Verification items for the finished model (mm, model axes). A direction names the side the tool comes from. Round coordinates to 2 decimals unless told otherwise and drop trailing zeros. Write each loop counter-clockwise with the first axis right and the second up, starting at its lowest first coordinate (ties: lowest second). Pieces come first, ordered by that corner, then holes. Notation, with made-up numbers: (89, 41.25) - (131, 41.25) arc R25 ccw to (131, 72.25) - close; hole circle Ø6 at (8.25, 53). An arc over 180 degrees is marked (long way). Write each question's results on one line, items separated by ' | '.
```python
from build123d import *

# Parameters (mm, degrees)
F0_R     = 5
F1_DEPTH = 78.5
F2_R     = 1.5
F3_DEPTH = 7


with BuildPart() as f1:
    # F0 (on Right) → F1 (new body)
    with BuildSketch(Plane.YZ):
        Circle(F0_R)
    extrude(amount=F1_DEPTH)

    # F2 (on face) → F3 (join)
    with BuildSketch(Plane.YZ.offset(78.5)):
        Circle(F2_R)
    extrude(amount=F3_DEPTH)

    # F4: F1 across plane


with BuildPart() as f1_1:
    add(f1.part)
    add(f1.part.mirror(Plane.YZ))


solid = f1_1.part
```
(1) Set-up check for faces 1 (the cylindrical face through (1.1, -1.08, -4.88)), 2 (the flat face through (78.5, -1.2, 1.2)), 3 (the cylindrical face through (-81.95, -1.5, 0.07)): record each of +Z, -Z, +X, -X, +Y, -Y from which the full face is reachable in a straight line by a thin tool's end or side.
Answer:
face 1: +X, -X | face 2: +X | face 3: -X
(2) Go/stop test with flat-tipped pins: pin 1 Ø2 at (x, z) = (19.5, 1.5) entering from -Y; pin 2 Ø1 at (x, y) = (-21, 3.5) entering from +Z; pin 3 Ø2 at (y, z) = (-0.5, 3.5) entering from +X. Record where each tip stops, or that it passes through.
Answer:
pin 1: y = -4.97 | pin 2: z = 4 | pin 3: x = 78.5
(3) Thickness scan on L1, parallel to Z at x = -5, y = 0.5; L2, parallel to X at y = -2, z = 1.5. Record the ranges inside material, lowest first.
Answer:
L1: -4.97 to 4.97 | L2: -78.5 to 78.5
(4) Section check A-A (z = 0). Record the cut outline in (x, y).
Answer:
outline: (-85.5, -1.5) - (-78.5, -1.5) - (-78.5, -5) - (78.5, -5) - (78.5, -1.5) - (85.5, -1.5) - (85.5, 1.5) - (78.5, 1.5) - (78.5, 5) - (-78.5, 5) - (-78.5, 1.5) - (-85.5, 1.5) - close
(5) Section check C-C (x = -3). Record the cut outline in (y, z), plus the area to 3 significant figures.
Answer:
outline: circle Ø10 at (0, 0) | area: 78.5 mm2
